Could you check a few things on this model? Use its own coordinates, in mm. Face numbers are marked on the shaded views. A direction names the side the tool comes from. Round coordinates to 2 decimals unless told otherwise and drop trailing zeros. Loops run counter-clockwise (first coordinate to the right, second up) from the corner with the lowest first, then second, coordinate; pieces in that order, holes last. Notation, with made-up numbers: M -14,79 L -9,79 A13 ccw -9,90 Z; hole C 79,23 d10. An arc over 180 degrees is marked long. One line per item, written item: value. Start each with the question number.
Q1. I'm going to push flat-ended pins straight in: pin 1 Ø1 at (x, z) = (3, 1) entering from -Y; pin 2 Ø0.8 at (y, z) = (8.5, 1) entering from +X; pin 3 Ø1 at (y, z) = (6.5, 0.5) entering from -X. Where does each tip first touch, or does it pass through?
Q2. Please list where these lines run through material, in increasing order: line 1 along X through (y, z) = (12.5, 0.2); line 2 along X through (y, z) = (8, 2.4); line 3 along X through (y, z) = (11.25, 2.3).
Q3. Which directions (+Z, -Z, +X, -X, +Y, -Y) give clear straight access to the entire face, cutting with the end or side of a thin tool? Please do the marked faces 5, 6 and 7.
Q4. Imagine slicing it at A-A (y = 7). Please give me the cut outline in (x, z).
Q5. Thinking about a two-plate mould opening in Y: for the marked faces 1, 2, 3 and 4, which applies, released by +Y, released by -Y, zero draft, split by the parting line, or undercut?
Q6. Imagine slicing it at B-B (x = 9.5). Please give me the cut outline in (y, z), then the cut area to 3 significant figures.
Q7. Imagine slicing it at D-D (z = 0.6). Please give me the cut outline in (x, y), then the cut area to 3 significant figures.
Q8. Imagine slicing it at C-C (y = 11.75). Please give me the cut outline in (x, z).
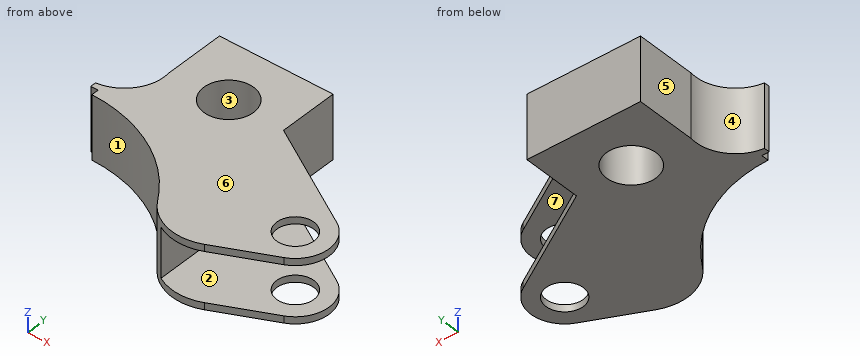
Autodesk Inventor part; units mm, degrees
ref_plane "Work Plane3" through (11.9729, 7.351, 2.56) normal (0.9986772, -0.0514186, 0) x (0.0514186, 0.9986772, 0)
ref_plane "YZ Plane" through (0, 0, 0) normal (1, 0, 0) x (0, 1, 0)
ref_plane "XZ Plane" through (0, 0, 0) normal (0, 1, 0) x (-1, 0, 0)
sketch "Sketch1" plane through (0, 0, 0) normal (0, 0, 1) x (1, 0, 0)
  line L0 (0, 0) -> (13.07, 0) construction
  line L1 (13.07, 0) -> (13.07, 20) construction
  line L2 (13.07, 20) -> (0, 20) construction
  line L3 (0, 20) -> (0, 0) construction
  line L4 (0.0102, 11.1339) -> (2.4902, 11.1339) construction
  line L5 (7.0502, 11.1097) -> (11.3067, 8.5922)
  arc A0 (11.1827, 6.1848) -> (11.3067, 8.5922) centre (10.614, 7.421) ccw
  line L6 (2.4702, 13.4954) -> (7.0502, 13.4953)
  line L7 (7.0502, 13.4953) -> (7.0502, 11.1097)
  line L8 (2.4702, 11.0654) -> (2.4702, 13.4954)
  circle A1 centre (4.7602, 11.2054) radius 1
  circle A2 centre (4.7602, 11.2054) radius 2.29 construction
  circle A3 centre (10.614, 7.421) radius 0.75
  line L9 (7.0502, 11.1097) -> (7.0502, 4.2834) construction
  line L10 (11.1827, 6.1848) -> (7.0502, 4.2834)
  arc A4 (1.0511, 9.2211) -> (2.4702, 11.0654) centre (0.8865, 10.8158) ccw
  line L11 (1.0511, 9.2211) -> (1.0511, 8.9911)
  line L12 (1.0511, 8.9911) -> (1.3499, 8.9911)
  line L13 (1.3499, 8.9911) -> (1.3499, 8.6911)
  arc A5 (7.0502, 4.2834) -> (1.3499, 8.6911) centre (1.2762, 2.706) ccw
  point P0 (0, 8.9921)
  point P1 (0, 7.8144)
  point P2 (0, 7.3623)
  dimension "d0" = 20
  dimension "d1" = 13.07
  dimension "d7" = 2
  dimension "d8" = 4.58
  dimension "d11" = 1.5
  dimension "d34" = 0.23
  dimension "d35" = 0.3
extrude "Extrusion2" add sketch "Sketch1" along normal blind 2.56
ref_plane "Work Plane3" through (11.9729, 7.351, 2.56) normal (0.9986772, -0.0514186, 0) x (0.0514186, 0.9986772, 0)
sketch "Sketch5" plane through (11.9729, 7.351, 2.56) normal (0.9986772, -0.0514186, 0) x (0.0514186, 0.9986772, 0)
  line L0 (3.5006, -2.56) -> (3.5006, 0)
  line L1 (3.5006, -1.28) -> (3.5006, -0.28)
  line L2 (3.5006, -0.28) -> (3.5006, -1.28)
  line L3 (3.5006, -1.28) -> (3.5006, -2.28)
  line L4 (3.5006, -0.28) -> (-3.2437, -0.28)
  line L5 (-3.2437, -0.28) -> (-3.2437, -2.28)
  line L6 (3.5006, -2.28) -> (-3.2437, -2.28)
  point P0 (-7.9569, -2.56)
  dimension "d29" = 1
  dimension "d30" = 1
extrude "Extrusion6" cut sketch "Sketch5" against normal up to surface surface through (7.0502, 11.1097, 0) normal (1, -0.000029, 0)
fillet "Fillet3" radius 2 1 edges at (7.0502, 4.2834, 1.28)
properties material "Liga de Nickel-Copper 400"
Report:
1. pin 1: stops at y = 8.26
1. pin 2: stops at x = 7.05
1. pin 3: stops at x = 5.45
2. line 1: x = 2.47 to 7.05
2. line 2: x = 4.07 to 10.14, 11.09 to 11.85
2. line 3: x = 2.47 to 3.76, 5.76 to 7.05
3. face 5: +Z, -Z, -X, +Y
3. face 6: +Z, +X, -X, +Y, -Y
3. face 7: +X, +Y, -Y
4. outline: M 5.45,0 L 9.99,0 L 9.99,0.28 L 7.05,0.28 L 7.05,2.28 L 9.99,2.28 L 9.99,2.56 L 5.45,2.56 Z; M 11.23,0 L 11.91,0 L 11.91,0.28 L 11.23,0.28 Z; M 11.23,2.28 L 11.91,2.28 L 11.91,2.56 L 11.23,2.56 Z
5. face 1: released by -Y
5. face 2: zero draft
5. face 3: undercut
5. face 4: undercut
6. outline: M 5.41,0 L 9.66,0 L 9.66,0.28 L 5.41,0.28 Z; M 5.41,2.28 L 9.66,2.28 L 9.66,2.56 L 5.41,2.56 Z
6. area: 2.38 mm²
7. outline: M 1.05,8.99 L 1.35,8.99 L 1.35,8.69 A5.99 cw 6.35,5.88 A2 ccw 7.05,5.21 L 7.05,13.5 L 2.47,13.5 L 2.47,11.07 A1.6 cw 1.05,9.22 Z; hole C 4.76,11.21 d2
7. area: 26.5 mm²
8. outline: M 2.47,0 L 3.92,0 L 3.92,2.56 L 2.47,2.56 Z; M 5.6,0 L 7.05,0 L 7.05,2.56 L 5.6,2.56 Z
